Read the model definition and answer for the solid it produces. Units are mm, in the model's axes. Face numbers are marked on the shaded views. Coordinates: 2 decimals unless noted, no trailing zeros. Order: outer loops, then holes, each group sorted by start corner. A loop starts at its lowest first (then second) coordinate and runs counter-clockwise, first axis right, second up. Notation, with made-up numbers: (-40, 48.5) -> (0, 48.5) arc R34 ccw to (0, 85.5) -> close; hole circle Ø5 at (49, 26.5). An arc over 180 degrees is marked (long way). Answer as a JSON object with one key per item and string values. Group by question number.
1) Determine the mould class of the marked faces 1, 2, 3 and 4 for opening direction Z: released by +Z, released by -Z, zero draft, split by the parting line, or undercut.
2) Section A-A on z = 0 is taken. Determine the outline of the cut face in (x, y), and give its area (3 significant figures).
3) Consider L1, parallel to X at y = -108, z = -73; L2, parallel to X at y = -43, z = -77.5; L3, parallel to Z at x = 298.5, y = -13.5. Determine where each line is inside the solid, lowest interval first.
4) Given pin 1 (5 mm diameter, centred on x = -460, y = -91, fed in from -Z); pin 2 (12 mm diameter, centred on x = 441, y = -33.5, fed in from +Z); pin 3 (10 mm diameter, centred on y = -63, z = 40.5, fed in from -X), each flat-ended and moving along its own axis, determine where each tip first touches the part or whether it passes through.
5) Section B-B on x = 478 is taken. Determine the outline of the cut face in (y, z), and give its area (3 significant figures).
6) Section C-C on y = -22.5 is taken. Determine the outline of the cut face in (x, z), and give its area (3 significant figures).
7) Section D-D on z = -58 is taken. Determine the outline of the cut face in (x, y).
from build123d import *

# Parameters (mm, degrees)
F0_R     = 101.6
F1_DEPTH = 127


with BuildPart() as f1:
    # F0 (on Front) → F1 (new body)
    with BuildSketch(Plane.XZ):
        with BuildLine():
            ThreePointArc((-350.5727146354, -249.7614733395), (-177.0893178173, -174.9104050294), (-105.6363849792, 0))
            ThreePointArc((-105.6363849792, 0), (-177.6708286975, 175.5014063187), (-352.230732019, 249.7883153539))
            ThreePointArc((-352.230732019, 249.7883153539), (-605.2222561445, 4.0063838927), (-360.2434595529, -249.7629175066))
            Line((-360.2434595529, -249.7629175066), (-350.5727146354, -249.7614733395))
        make_face()
        with Locations((-355.4453849792, 0)):
            Circle(F0_R, mode=Mode.SUBTRACT)
        with BuildLine():
            ThreePointArc((-352.230732019, 249.7883153539), (-177.6708286975, 175.5014063187), (-105.6363849792, 0))
            Line((-105.6363849792, 0), (157.0365696106, 0))
            ThreePointArc((157.0365696106, 0), (228.6283631182, 175.0518888532), (402.3693141559, 249.7688924148))
            Line((402.3693141559, 249.7688924148), (-352.230732019, 249.7883153539))
        make_face()
        with BuildLine():
            Line((157.0365696106, 0), (-105.6363849792, 0))
            ThreePointArc((-105.6363849792, 0), (-177.0893178173, -174.9104050294), (-350.5727146354, -249.7614733395))
            Line((-350.5727146354, -249.7614733395), (397.9256440217, -249.6496973931))
            ThreePointArc((397.9256440217, -249.6496973931), (227.0779221147, -173.4593018399), (157.0365696106, 0))
        make_face()
        with BuildLine():
            ThreePointArc((402.3693141559, 249.7688924148), (228.6283631182, 175.0518888532), (157.0365696106, 0))
            ThreePointArc((157.0365696106, 0), (227.0779221147, -173.4593018399), (397.9256440217, -249.6496973931))
            Line((397.9256440217, -249.6496973931), (415.8400569706, -249.6470221696))
            ThreePointArc((415.8400569706, -249.6470221696), (586.6391184019, -173.4324545581), (656.6545696106, 0))
            ThreePointArc((656.6545696106, 0), (581.8974584638, 178.2172064924), (402.3693141559, 249.7688924148))
        make_face()
        with BuildLine():
            ThreePointArc((509.2094031334, 0), (407.6094031334, -101.6), (306.0094031334, 0))
            ThreePointArc((306.0094031334, 0), (407.6094031334, 101.6), (509.2094031334, 0))
        make_face(mode=Mode.SUBTRACT)
        with BuildLine():
            ThreePointArc((-360.2434595529, -249.7629175066), (-355.4080801051, -249.8089972146), (-350.5727146354, -249.7614733395))
            Line((-350.5727146354, -249.7614733395), (-360.2434595529, -249.7629175066))
        make_face()
        with BuildLine():
            Line((415.8400569706, -249.6470221696), (397.9256440217, -249.6496973931))
            ThreePointArc((397.9256440217, -249.6496973931), (406.8828744847, -249.8089972146), (415.8400569706, -249.6470221696))
        make_face()
    extrude(amount=F1_DEPTH)


solid = f1.part
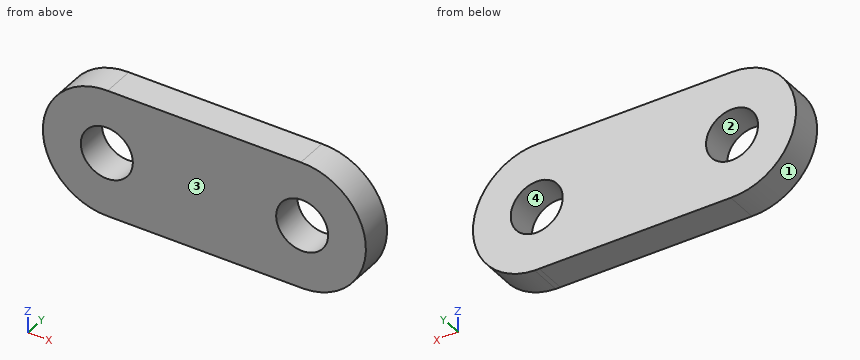
Worked answers:
{
 "1": {"face 1": "split by the parting line", "face 2": "undercut", "face 3": "zero draft", "face 4": "undercut"},
 "2": {"outline": "(-605.25, -127) -> (-457.05, -127) -> (-457.05, 0) -> (-605.25, 0) -> close; (-253.85, -127) -> (306.01, -127) -> (306.01, 0) -> (-253.85, 0) -> close; (509.21, -127) -> (656.65, -127) -> (656.65, 0) -> (509.21, 0) -> close", "area": "109,000 mm²"},
 "3": {"L1": "x = -594.35 to -426.11, -284.78 to 336.94, 478.27 to 645.75", "L2": "x = -592.93 to -421.14, -289.75 to 341.91, 473.31 to 644.33", "L3": "z = -249.66 to 249.77"},
 "4": {"pin 1": "stops at z = -228.01", "pin 2": "stops at z = 248.22", "pin 3": "stops at x = -602.72"},
 "5": {"outline": "(-127, -239.46) -> (0, -239.46) -> (0, -73.26) -> (-127, -73.26) -> close; (-127, 73.26) -> (0, 73.26) -> (0, 239.46) -> (-127, 239.46) -> close", "area": "42,200 mm²"},
 "6": {"outline": "(-352.23, 249.79) arc R249.81 ccw (long way) to (-350.57, -249.76) -> (397.93, -249.65) arc R249.81 ccw (long way) to (402.37, 249.77) -> close; hole circle Ø203.2 at (-355.45, 0); hole circle Ø203.2 at (407.61, 0)", "area": "512,000 mm²"},
 "7": {"outline": "(-598.43, -127) -> (-438.86, -127) -> (-438.86, 0) -> (-598.43, 0) -> close; (-272.03, -127) -> (324.19, -127) -> (324.19, 0) -> (-272.03, 0) -> close; (491.03, -127) -> (649.83, -127) -> (649.83, 0) -> (491.03, 0) -> close"}
}
